from build123d import *

# Parameters (mm, degrees)
SKETCH_1_R      = 5.7
EXTRUDE_1_DEPTH = 1.3
EXTRUDE_2_DEPTH = 2.8
EXTRUDE_3_DEPTH = 0.2
EXTRUDE_4_DEPTH = 0.4


with BuildPart() as part:
    # Эскиз1 → Бобышка-Вытянуть1 (new body)
    with BuildSketch(Plane.XY):
        Circle(SKETCH_1_R)
    extrude(amount=EXTRUDE_1_DEPTH)

    # Эскиз2 → Бобышка-Вытянуть2 (add)
    with BuildSketch(Plane.XY.offset(1.3)):
        with BuildLine():
            Line((-2.5, 6.5), (2.5, 6.5))
            ThreePointArc((2.5, 6.5), (9, 0), (2.5, -6.5))
            Line((2.5, -6.5), (-2.5, -6.5))
            ThreePointArc((-2.5, -6.5), (-9, 0), (-2.5, 6.5))
        make_face()
    extrude(amount=EXTRUDE_2_DEPTH)

    # Эскиз3 → Бобышка-Вытянуть3 (add)
    with BuildSketch(Plane.XY.offset(4.1)):
        with BuildLine():
            Line((-2.5, 6.5), (2.5, 6.5))
            ThreePointArc((2.5, 6.5), (9, 0), (2.5, -6.5))
            Line((2.5, -6.5), (-2.5, -6.5))
            ThreePointArc((-2.5, -6.5), (-9, 0), (-2.5, 6.5))
        make_face()
        with BuildLine():
            Line((-2.75, 4.5), (2.75, 4.5))
            ThreePointArc((2.75, 4.5), (7.25, 0), (2.75, -4.5))
            Line((2.75, -4.5), (-2.75, -4.5))
            ThreePointArc((-2.75, -4.5), (-7.25, 0), (-2.75, 4.5))
        make_face(mode=Mode.SUBTRACT)
    extrude(amount=EXTRUDE_3_DEPTH)

    # Эскиз4 → Бобышка-Вытянуть4 (add)
    with BuildSketch(Plane(origin=(0, 0, 1.3), x_dir=(-1, 0, 0), z_dir=(0, 0, -1))):
        with BuildLine():
            Line((5.355682571, 2.5), (8.331941275, 2.5))
            ThreePointArc((8.331941275, 2.5), (7.241539509, 4.216555717), (5.664101615, 5.5))
            Line((5.664101615, 5.5), (2.164101615, 5.5))
            ThreePointArc((2.164101615, 5.5), (4.04805985, 4.306570242), (5.355682571, 2.5))
        make_face()
        with BuildLine():
            Line((5.355682571, -2.5), (8.331941275, -2.5))
            ThreePointArc((8.331941275, -2.5), (7.241539509, -4.216555717), (5.664101615, -5.5))
            Line((5.664101615, -5.5), (2.164101615, -5.5))
            ThreePointArc((2.164101615, -5.5), (4.04805985, -4.306570242), (5.355682571, -2.5))
        make_face()
    extrude(amount=EXTRUDE_4_DEPTH)


solid = part.part
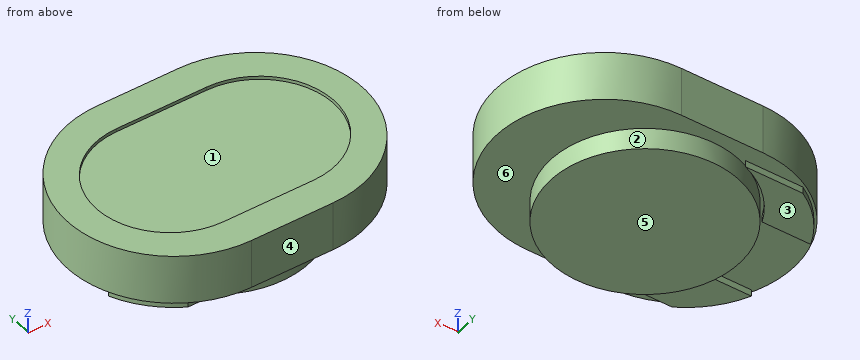
Check sheet for the modelled part. Datum: model origin and axes. Units: mm. Face numbers are marked on the shaded views. A direction names the side the tool comes from. Give positions to 0.01 mm unless a question says otherwise; leave off trailing zeros. Order: outer loops, then holes, each group sorted by start corner. A loop starts at its lowest first (then second) coordinate and runs counter-clockwise, first axis right, second up. Notation, with made-up numbers: M 0,-28.75 L 59,-28.75 A24 cw 59,-8.75 Z; hole C 57.5,55.25 d1. An arc over 180 degrees is marked long. Answer as CSV lines item,"result". Start each with the question number.
Item 1: Cross-section at B-B on y = 0. Enter the section's corners in (x, z), plus the area to 3 significant figures.
Item 2: Gauge pin test, flat ends, axial feed: P1, Ø0.9, axis at x = -6.5, y = 4.5, coming from the -Z side; P2, Ø6.5, axis at x = 3.5, y = 3, coming from the -Z side; P3, Ø1, axis at x = 5.5, y = -3, coming from the -Z side; P4, Ø4.5, axis at x = -3, y = 1, coming from the +Z side. Record the tip position at first contact, or that the pin passes through.
Item 3: Tool access check on the marked faces 1, 2 and 3. Record the directions out of +Z, -Z, +X, -X, +Y, -Y that give a thin tool (end or side, any length) a straight path to the whole face; none if there is none.
Item 4: Cross-section at A-A on x = 0. Enter the section's corners in (y, z), plus the area to 3 significant figures.
Item 5: Thickness scan on line 1 (Z direction, x = 4, y = -1.25); line 2 (Z direction, x = 3, y = 5); line 3 (X direction, y = 1.5, z = 0.3). Record the ranges inside material, lowest first. Write a range as [from, to].
Item 6: Cross-section at C-C on z = 0.4. Enter the section's corners in (x, y), plus the area to 3 significant figures.
Item 7: Mould release check, pull along Y, two halves, no side actions. Record for the marked faces 4, 5 and 6: +Y half, -Y half, draft (parallel to the pull), parting line (faces both ways), or undercut.
Item 8: Cross-section at D-D on x = -4. Enter the section's corners in (y, z).
Established:
1,outline,"M -9,1.3 L -5.7,1.3 L -5.7,0 L 5.7,0 L 5.7,1.3 L 9,1.3 L 9,4.3 L 7.25,4.3 L 7.25,4.1 L -7.25,4.1 L -7.25,4.3 L -9,4.3 Z"
1,area,"65.9 mm^2"
2,P1,"stops at z = 0.9"
2,P2,"stops at z = 0"
2,P3,"stops at z = 1.3"
2,P4,"stops at z = 4.1"
3,face 1,"+Z"
3,face 2,"-Z"
3,face 3,"-Z, -X, +Y"
4,outline,"M -6.5,1.3 L -5.7,1.3 L -5.7,0 L 5.7,0 L 5.7,1.3 L 6.5,1.3 L 6.5,4.3 L 4.5,4.3 L 4.5,4.1 L -4.5,4.1 L -4.5,4.3 L -6.5,4.3 Z"
4,area,"52.0 mm^2"
5,line 1,"z = [0, 4.1]"
5,line 2,"z = [1.3, 4.3]"
5,line 3,"x = [-5.5, 5.5]"
6,outline,"C 0,0 d11.4"
6,area,"102 mm^2"
7,face 4,"-Y half"
7,face 5,"draft"
7,face 6,"undercut"
8,outline,"M -6.32,1.3 L -5.5,1.3 L -5.5,0.9 L -4.35,0.9 L -4.35,1.3 L -4.06,1.3 L -4.06,0 L 4.06,0 L 4.06,1.3 L 4.35,1.3 L 4.35,0.9 L 5.5,0.9 L 5.5,1.3 L 6.32,1.3 L 6.32,4.3 L 4.32,4.3 L 4.32,4.1 L -4.32,4.1 L -4.32,4.3 L -6.32,4.3 Z"
